Answer from the drawing. Dimensions are ordinates in mm from the lowest x, y and z of the part. Give positions to 0.01 mm unless a question says otherwise; leave off trailing zeros. Loops run counter-clockwise (first coordinate to the right, second up) from the corner with the lowest first, then second, coordinate; pieces in that order, holes last. Notation, with made-up numbers: M 84.25,88 L 112.25,88 A19 ccw 112.25,107 Z; hole C -1,62 d2. An arc over 180 degrees is marked long. Use a Markdown table: item, result.
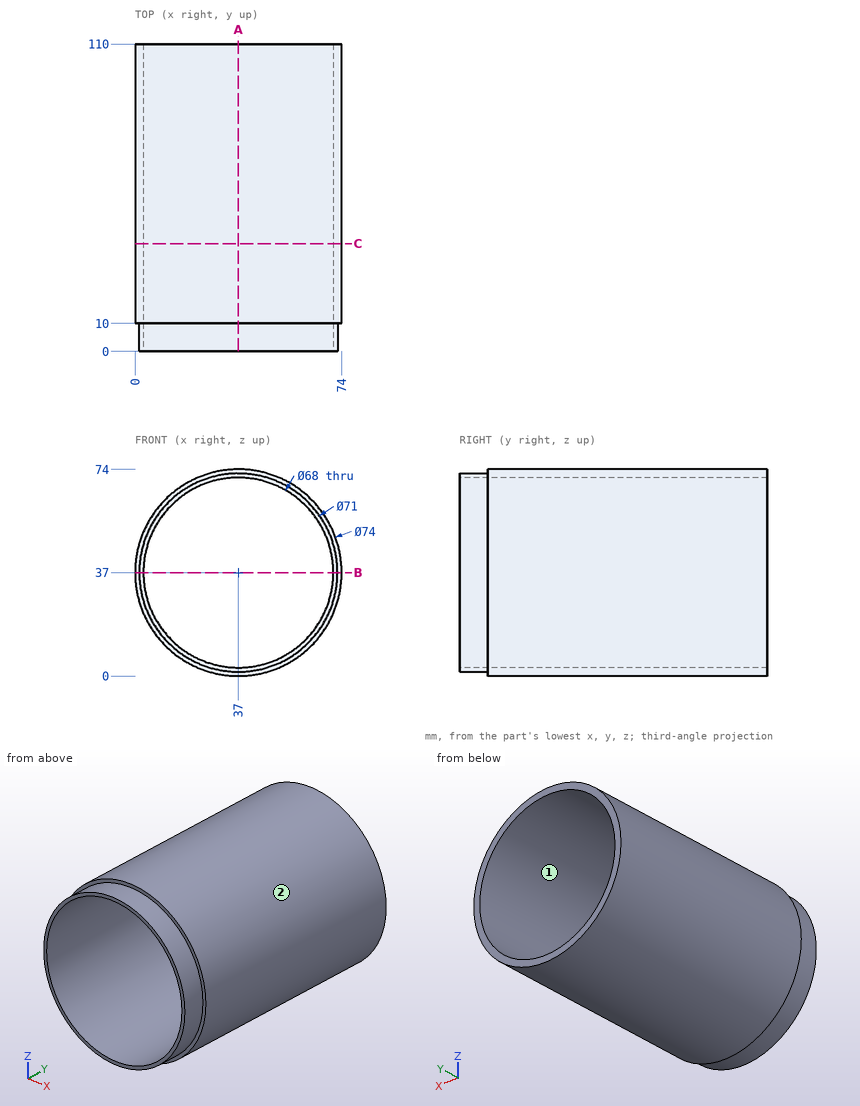
(1) Given P1, Ø1, axis at y = 89, z = 60, coming from the -X side; P2, Ø3, axis at x = 15.5, y = 95.5, coming from the +Z side; P3, Ø2, axis at x = 63.5, y = 37.5, coming from the +Z side, each flat-ended and moving along its own axis, determine where each tip first touches the part or whether it passes through.
Entries:
| item | result |
|---|---|
| P1 | stops at x = 7.63 |
| P2 | stops at z = 68.13 |
| P3 | stops at z = 63.81 |
(2) A cutting plane is placed at C-C (y = 38.5). Write down the section's boundary in (x, z).
Entries:
| item | result |
|---|---|
| outline | C 37,37 d74; hole C 37,37 d68 |
(3) Consider probe 1 along Z at (x, y) = (37, 52); probe 2 along X at (y, z) = (25, 11). Determine where each line is inside the solid, lowest interval first. Write a range as [from, to].
Entries:
| item | result |
|---|---|
| probe 1 | z = [0, 3], [71, 74] |
| probe 2 | x = [10.68, 15.09], [58.91, 63.32] |
(4) The mould has two halves that part along X. Classify the marked faces 1 and 2: released by +X, released by -X, zero draft, split by the parting line, or undercut.
Entries:
| item | result |
|---|---|
| face 1 | undercut |
| face 2 | split by the parting line |
(5) A cutting plane is placed at B-B (z = 37). Write down the section's boundary in (x, y), and give its area (3 significant figures).
Entries:
| item | result |
|---|---|
| outline | M 0,10 L 1.5,10 L 1.5,0 L 3,0 L 3,110 L 0,110 Z; M 71,0 L 72.5,0 L 72.5,10 L 74,10 L 74,110 L 71,110 Z |
| area | 630 mm² |
(6) A cutting plane is placed at A-A (x = 37). Write down the section's boundary in (y, z), and give its area (3 significant figures).
Entries:
| item | result |
|---|---|
| outline | M 0,1.5 L 10,1.5 L 10,0 L 110,0 L 110,3 L 0,3 Z; M 0,71 L 110,71 L 110,74 L 10,74 L 10,72.5 L 0,72.5 Z |
| area | 630 mm² |
